Input: part model. Units: mm. Frame: model coordinates. A direction names the side the tool comes from. Coordinates: 2 decimals unless noted, no trailing zeros. Write each loop counter-clockwise with the first axis right and the second up, starting at its lowest first coordinate (ties: lowest second). Pieces come first, ordered by that corner, then holes. Notation, with made-up numbers: (22, 12.25) - (48, 12.25) arc R23 cw to (48, 45.25) - close; hole circle Ø8 at (12, 53.5). An arc over 180 degrees is marked (long way). Use CSV: the item, a comma, the result in double quotes.
```python
from build123d import *

# Parameters (mm, degrees)
CHAMFER1_SIZE = 1


with BuildPart() as part:
    # Sketch1 → Revolve1 (revolve)
    with BuildSketch(Plane.XY):
        Polygon((0, 22.5), (0, 42.5), (22, 42.5), (22, 28.5), (41.5, 28.5), (41.5, 22.5), align=None)
    revolve(axis=Axis((43.575, 0, 0), (-1, 0, 0)))

    # Chamfer1
    chamfer1_edges = [part.edges().sort_by_distance(p)[0] for p in [
        (0, -42.5, 0),
        (0, -22.5, 0),
        (41.5, -22.5, 0),
        (41.5, -28.5, 0),
        (22, -28.5, 0),
        (22, -42.5, 0),
    ]]
    chamfer(chamfer1_edges, length=CHAMFER1_SIZE)


solid = part.part
```
(1) Reachability of faces 4 (the cylindrical face through (31.873, 26.327, 10.916)), 5 (the flat face through (41.5, 20.2, -12.4)) from +Z, -Z, +X, -X, +Y, -Y: full face, straight path, thin tool, end or side. Return the list, or none.
Check values:
face 4,"+X"
face 5,"+Z, -Z, +X, +Y, -Y"
(2) Ray query, probe 1 along Y at (x, z) = (17, 0); probe 2 along Y at (x, z) = (25.5, 0). Return the intervals inside material, ascending. Write a range as from..to.
Check values:
probe 1,"-42.5..-22.5, 22.5..42.5"
probe 2,"-28.5..-22.5, 22.5..28.5"
(3) Cut plane D-D on x = 6.5. Return loops of the section in (y, z).
Check values:
outline,"circle Ø85 at (0, 0); hole circle Ø45 at (0, 0)"
(4) Draft query along Z for faces 1 (the cylindrical face through (11.14, -33.727, 25.861)), 2 (the cylindrical face through (20.474, 10.382, 19.961)), 3 (the flat face through (22, -10, -28)). Return one class per face: pulls with the +Z half, pulls with the -Z half, needs draft (parallel to the pull), parting line crosses it, or undercut.
Check values:
face 1,"parting line crosses it"
face 2,"undercut"
face 3,"needs draft"
(5) Cut plane A-A on y = 0. Return loops of the section in (x, z), and give its area (3 significant figures).
Check values:
outline,"(0, -41.5) - (1, -42.5) - (21, -42.5) - (22, -41.5) - (22, -29.5) - (23, -28.5) - (40.5, -28.5) - (41.5, -27.5) - (41.5, -23.5) - (40.5, -22.5) - (1, -22.5) - (0, -23.5) - close; (0, 23.5) - (1, 22.5) - (40.5, 22.5) - (41.5, 23.5) - (41.5, 27.5) - (40.5, 28.5) - (23, 28.5) - (22, 29.5) - (22, 41.5) - (21, 42.5) - (1, 42.5) - (0, 41.5) - close"
area,"1,110 mm^2"
(6) Pin query (flat end, axial travel): pin 1 Ø3 at (x, z) = (20, 14) entering from +Y; pin 2 Ø2 at (x, y) = (12, -27) entering from +Z; pin 3 Ø3 at (x, y) = (8.5, -12.5) entering from -Z. Return the tip coordinate at first contact, or that it passes through.
Check values:
pin 1,"y = 40.62"
pin 2,"z = 33.62"
pin 3,"z = -41.05"
(7) Cut plane C-C on x = 30. Return loops of the section in (y, z).
Check values:
outline,"circle Ø57 at (0, 0); hole circle Ø45 at (0, 0)"
